Read the model definition and answer for the solid it produces. Units are mm, in the model's axes. A direction names the side the tool comes from. Coordinates: 2 decimals unless noted, no trailing zeros. Loops run counter-clockwise (first coordinate to the right, second up) from the corner with the lowest first, then second, coordinate; pieces in that order, holes last. Notation, with made-up numbers: M -22,-11 L -13,-11 A17 ccw -13,11 Z; hole C 55,85 d8. An arc over 180 degrees is marked long. One line per item, written item: value. Start each with the question number.
1. Determine the mould class of faces 1 (the face through (-0.1, 12.5, -4.3)), 2 (the face through (0, -0.5, 0)), 3 (the face through (-2.17, -0.18, -9.76)) for opening direction X: +X half, -X half, draft (parallel to the pull), parting line (faces both ways), or undercut.
2. Flat-ended cylindrical pins translate along their axes: pin 1 (3 mm diameter, centred on y = 3.5, z = 3.5, fed in from -X); pin 2 (2.5 mm diameter, centred on x = -1.5, z = 1, fed in from +Y); pin 3 (12 mm diameter, centred on x = -7.5, y = -4, fed in from -Z). Find the tip coordinate at first contact, or state that the pin passes through.
3. The part is cut by section B-B (z = 0). Write down the section's boundary in (x, y), then the cut area to 3 significant figures.
4. For faces 4 (the face through (-0.54, -6.58, -2.44)), 5 (the face through (0, 0.5, 0)), 6 (the face through (2, -12.5, -2)), determine the directions among +Z, -Z, +X, -X, +Y, -Y from which every point of the face is accessible in a straight line to the end or side of a thin tool.
5. The part is cut by section C-C (x = 0). Write down the section's boundary in (y, z), then the cut area to 3 significant figures.
6. The part is cut by section A-A (y = -10.25). Write down the section's boundary in (x, z), then the cut area to 3 significant figures.
7. Consider probe 1 along Z at (x, y) = (0, -9.75); probe 2 along Z at (x, y) = (0, 6.5); probe 3 along X at (y, z) = (-8.75, 1.75). Determine where each line is inside the solid, lowest interval first.
8. The part is cut by section D-D (y = 9.75). Write down the section's boundary in (x, z).
```python
from build123d import *

# Parameters (mm, degrees)
F0_R     = 10
F1_DEPTH = 12.5
F2_R     = 2.5
F3_DEPTH = 12
F4_R     = 4
F5_DEPTH = 12


with BuildPart() as f1:
    # F0 (on Front) → F1 (new body, symmetric)
    with BuildSketch(Plane.XZ):
        Circle(F0_R)
    extrude(amount=F1_DEPTH, both=True)

    # F2 (on face) → F3 (cut)
    with BuildSketch(Plane.XZ.offset(12.5)):
        Circle(F2_R)
    extrude(amount=-F3_DEPTH, mode=Mode.SUBTRACT)

    # F4 (on face) → F5 (cut)
    with BuildSketch(Plane(origin=(0, 12.5, 0), x_dir=(-1, 0, 0), z_dir=(0, 1, 0))):
        Circle(F4_R)
    extrude(amount=-F5_DEPTH, mode=Mode.SUBTRACT)


solid = f1.part
```
Answer block:
1. face 1: draft
1. face 2: undercut
1. face 3: parting line
2. pin 1: stops at x = -9.8
2. pin 2: stops at y = 0.5
2. pin 3: stops at z = -9.89
3. outline: M -10,-12.5 L -2.5,-12.5 L -2.5,-0.5 L 2.5,-0.5 L 2.5,-12.5 L 10,-12.5 L 10,12.5 L 4,12.5 L 4,0.5 L -4,0.5 L -4,12.5 L -10,12.5 Z
3. area: 344 mm2
4. face 4: -Y
4. face 5: +Y
4. face 6: +Z, -Z, +X, -X, -Y
5. outline: M -12.5,-10 L 12.5,-10 L 12.5,-4 L 0.5,-4 L 0.5,4 L 12.5,4 L 12.5,10 L -12.5,10 L -12.5,2.5 L -0.5,2.5 L -0.5,-2.5 L -12.5,-2.5 Z
5. area: 344 mm2
6. outline: C 0,0 d20; hole C 0,0 d5
6. area: 295 mm2
7. probe 1: z = -10 to -2.5, 2.5 to 10
7. probe 2: z = -10 to -4, 4 to 10
7. probe 3: x = -9.85 to -1.79, 1.79 to 9.85
8. outline: C 0,0 d20; hole C 0,0 d8
